from build123d import *

# Parameters (mm, degrees)
CEK_ICECEK_ON_PU_37_5_1_START = 1
SKETCH1_W                     = 618
SKETCH1_H                     = 118
CEK_ICECEK_ON_PU_37_5_1_DEPTH = 37.5
CEK_ICECEK_ON_PU_37_5_2_START = 27
SKETCH2_W                     = 300
SKETCH2_H                     = 34
CEK_ICECEK_ON_PU_37_5_2_DEPTH = 14


with BuildPart() as part:
    # Sketch1 → CEK_icecek_on_pu_37.5_1 (new body)
    with BuildSketch(Plane.XY.offset(CEK_ICECEK_ON_PU_37_5_1_START)):
        with Locations((309, 59)):
            Rectangle(SKETCH1_W, SKETCH1_H)
    extrude(amount=CEK_ICECEK_ON_PU_37_5_1_DEPTH)

    # Sketch2 → CEK_icecek_on_pu_37.5_2 (cut)
    with BuildSketch(Plane.XY.offset(CEK_ICECEK_ON_PU_37_5_2_START)):
        with Locations((309, 75)):
            Rectangle(SKETCH2_W, SKETCH2_H)
    extrude(amount=CEK_ICECEK_ON_PU_37_5_2_DEPTH, mode=Mode.SUBTRACT)


solid = part.part
Source: CAD feature listing. Evaluate the final solid. Frame: model axes, mm. A direction names the side the tool comes from. Give positions to 0.01 mm unless a question says otherwise; leave off trailing zeros. Order: outer loops, then holes, each group sorted by start corner. A loop starts at its lowest first (then second) coordinate and runs counter-clockwise, first axis right, second up. Notation, with made-up numbers: (-26, 86) -> (-10, 86) arc R19 ccw to (-10, 103) -> close; hole circle Ø4 at (73, 82.5). An arc over 180 degrees is marked (long way). Use a Markdown table: item, result.
1) Reachability of faces 4 (the flat face through (307, 58, 33)), 5 (the flat face through (305, 60, 1)) from +Z, -Z, +X, -X, +Y, -Y: full face, straight path, thin tool, end or side. Return the list, or none.
Answer list:
| item | result |
|---|---|
| face 4 | +Z |
| face 5 | -Z, +X, -X, +Y, -Y |
2) Mould query, pull axis X, two halves, no side actions, for faces 1 (the flat face through (305, 47, 38.5)), 2 (the flat face through (0, 58, 19)), 3 (the flat face through (307, 92, 33)). Classes: +X half, -X half, draft (parallel to the pull), parting line (faces both ways), or undercut.
Answer list:
| item | result |
|---|---|
| face 1 | draft |
| face 2 | -X half |
| face 3 | undercut |
3) Section query B-B, the plane y = 80. Return the cut outline in (x, z).
Answer list:
| item | result |
|---|---|
| outline | (0, 1) -> (618, 1) -> (618, 38.5) -> (459, 38.5) -> (459, 27) -> (159, 27) -> (159, 38.5) -> (0, 38.5) -> close |
4) Section query A-A, the plane x = 168.5. Return the cut outline in (y, z), then the cut area to 3 significant figures.
Answer list:
| item | result |
|---|---|
| outline | (0, 1) -> (118, 1) -> (118, 38.5) -> (92, 38.5) -> (92, 27) -> (58, 27) -> (58, 38.5) -> (0, 38.5) -> close |
| area | 4,030 mm² |
5) Ray query, line 1 along Y through (x, z) = (207, 34); line 2 along X through (y, z) = (79, 35.5); line 3 along Z through (x, y) = (344, 85). Return the intervals inside material, ascending. Write a range as [from, to].
Answer list:
| item | result |
|---|---|
| line 1 | [0, 58], [92, 118] |
| line 2 | [0, 159], [459, 618] |
| line 3 | [1, 27] |
6) Contact query for flat-ended pins moving along their axis: P1, Ø12, axis at x = 250.5, z = 33, coming from the -Y side; P2, Ø17, axis at x = 361, y = 78, coming from the +Z side. Output: stop coordinate, or through.
Answer list:
| item | result |
|---|---|
| P1 | y = 0 |
| P2 | z = 27 |
